Work out the finished part from the listing and answer in its coordinate system (mm). A direction names the side the tool comes from. Coordinates: 2 decimals unless noted, no trailing zeros. Order: outer loops, then holes, each group sorted by start corner. A loop starts at its lowest first (then second) coordinate and runs counter-clockwise, first axis right, second up. Notation, with made-up numbers: M -38,-40 L -27,-40 A6 ccw -27,-31 Z; hole C 60,17 d1. An arc over 180 degrees is marked long. Write item = value, one per line. Start each with the question number.
Q1. Each of these flat-tipped pins is pushed along its axis until it touches: P1, Ø6, axis at x = -25.5, y = 60, coming from the -Z side; P2, Ø3, axis at y = 65.5, z = 7, coming from the -X side; P3, Ø5, axis at y = 123.5, z = 18, coming from the -X side; P4, Ø5, axis at y = 130, z = 4, coming from the +X side. Where does it stop, or does it pass through?
Q2. Find section C-C on x = -15.5. Give the vertices of the cut face in (y, z).
Q3. Find section B-B on y = 122.5. Give the vertices of the cut face in (x, z), and give its area (3 significant figures).
Q4. Straight lines are drawn through the part: line 1 along X through (y, z) = (127, 10); line 2 along Y through (x, z) = (-24, 9); line 3 along X through (y, z) = (125, 8.75). For each, find the intervals that lie inside material, in ascending order.
Q5. Determine the mould class of faces 6 (the flat face through (-37, 94, 25)), 7 (the cylindrical face through (-18.864, 45.315, 12.675)), 8 (the cylindrical face through (-46.17, 166.79, 12.32)), 9 (the cylindrical face through (-56.1, 155.8, 12.3)) for opening direction Y: released by +Y, released by -Y, zero draft, split by the parting line, or undercut.
Q6. A tool of negligible diameter and unlimited length cuts with its end or side. For faces 1 (the flat face through (-36.758, 121.268, 12.325)), 2 (the flat face through (-37.59, 57.57, 12.32)), 3 (the flat face through (-45.76, 86.6, 12.32)), 4 (the flat face through (-33.834, 78, 12)), 5 (the flat face through (-37, 94, 0)), from which of +Z, -Z, +X, -X, +Y, -Y can it reach the whole face along a straight path? Write none if from no direction.
```python
from build123d import *

# Parameters (mm, degrees)
F1_DEPTH  = 25
F2_DEPTH  = 25
F3_R      = 10.0351609687
F4_DEPTH  = 25
F5_W      = 5.021744368
F5_H      = 8.4
F5_W_2    = 5.524914672
F5_H_2    = 8.3
F6_DEPTH  = 28.7
F7_DEPTH  = 31.3
F8_W      = 20.0703219374
F8_H      = 8.3
F8_H_2    = 8.4
F9_DEPTH  = 25
F10_D     = 15
F11_DEPTH = 3
F12_DEPTH = 3
F13_DEPTH = 0.4
F15_DEPTH = 25
F16_R     = 5
F17_R     = 5
F18_R     = 5
F20_DEPTH = 25
F21_R     = 1
F22_DEPTH = 25
F24_DEPTH = 25
F25_R     = 2


with BuildPart() as f1:
    # F0 (on Top) → F1 (new body)
    with BuildSketch(Plane.XY):
        with BuildLine():
            Line((-46.5458918775, 92.7124905365), (-33.8341578848, 67.7643078592))
            Line((-33.8341578848, 67.7643078592), (-33.8341578848, 87.7643078592))
            Line((-33.8341578848, 87.7643078592), (-39.0436032148, 117.3085404495))
            ThreePointArc((-39.0436032148, 117.3085404495), (-50.1493049738, 127.7523979683), (-56.0863416463, 141.7938497088))
            Line((-56.0863416463, 141.7938497088), (-46.5458918775, 92.7124905365))
        make_face()
        Polygon((-26.4959632117, 42.4024048078), (0, 0), (0, 10), (-23.8463668905, 48.162164327), (-33.8341578848, 67.7643078592), (-46.5458918775, 92.7124905365), (-44.6555832012, 78.0426657754), align=None)
    extrude(amount=F1_DEPTH)

    # F0 (on Top) → F2 (join)
    with BuildSketch(Plane.XY):
        Polygon((-26.4959632117, 42.4024048078), (0, 0), (0, 10), (-23.8463668905, 48.162164327), (-33.8341578848, 67.7643078592), (-46.5458918775, 92.7124905365), (-44.6555832012, 78.0426657754), align=None)
        with BuildLine():
            Line((-46.5458918775, 92.7124905365), (-33.8341578848, 67.7643078592))
            Line((-33.8341578848, 67.7643078592), (-33.8341578848, 87.7643078592))
            Line((-33.8341578848, 87.7643078592), (-39.0436032148, 117.3085404495))
            ThreePointArc((-39.0436032148, 117.3085404495), (-50.1493049738, 127.7523979683), (-56.0863416463, 141.7938497088))
            Line((-56.0863416463, 141.7938497088), (-46.5458918775, 92.7124905365))
        make_face()
        with BuildLine():
            ThreePointArc((-51.0571508097, 168.5508889923), (-56.1292788842, 155.6530772369), (-56.0863416463, 141.7938497088))
            ThreePointArc((-56.0863416463, 141.7938497088), (-50.1493049738, 127.7523979683), (-39.0436032148, 117.3085404495))
            ThreePointArc((-39.0436032148, 117.3085404495), (-37.3018340244, 121.656861024), (-34.4069625383, 125.3394376776))
            ThreePointArc((-34.4069625383, 125.3394376776), (-34.1290622054, 125.5985630521), (-33.8452613454, 125.8512122687))
            ThreePointArc((-33.8452613454, 125.8512122687), (-46.0977457681, 142.6841841118), (-42.6035759811, 163.2088788258))
            ThreePointArc((-42.6035759811, 163.2088788258), (-46.2302574516, 166.8295340113), (-51.0571508097, 168.5508889923))
        make_face()
        with BuildLine():
            ThreePointArc((-34.4069625383, 125.3394376776), (-37.3018340244, 121.656861024), (-39.0436032148, 117.3085404495))
            Line((-39.0436032148, 117.3085404495), (-34.4069625383, 125.3394376776))
        make_face()
        with BuildLine():
            ThreePointArc((-46.2700698118, 143.7019396626), (-46.3013690244, 153.8058664235), (-42.6035759811, 163.2088788258))
            ThreePointArc((-42.6035759811, 163.2088788258), (-46.0977457681, 142.6841841118), (-33.8452613454, 125.8512122687))
            ThreePointArc((-33.8452613454, 125.8512122687), (-41.9417428936, 133.4651840398), (-46.2700698118, 143.7019396626))
        make_face()
    extrude(amount=F2_DEPTH)

    # F3 (on Top) → F4 (join)
    with BuildSketch(Plane.XY):
        Circle(F3_R)
    extrude(amount=F4_DEPTH)

    # F5 (on face) → F6 (join)
    with BuildSketch(Plane(origin=(0, 0, 0), x_dir=(0.5299192642, -0.8480480962, 0), z_dir=(-0.8480480962, -0.5299192642, 0))):
        with Locations((-12.5460331527, 4.2)):
            Rectangle(F5_W, F5_H)
        with Locations((-12.7976183047, 20.85)):
            Rectangle(F5_W_2, F5_H_2)
    extrude(amount=F6_DEPTH)

    # F7 (cut, symmetric): faces of the model
    f7_faces = [f1.faces().sort_by_distance(p)[0] for p in [
        (-17.4873152969, 0.9059577124, 20.85),
        (-17.4873152969, 0.9059577124, 4.2),
    ]]
    extrude(f7_faces, amount=F7_DEPTH, both=True, mode=Mode.SUBTRACT)

    # F8 (on face) → F9 (cut)
    with BuildSketch(Plane(origin=(0, 0, 0), x_dir=(0.5299192642, -0.8480480962, 0), z_dir=(-0.8480480962, -0.5299192642, 0))):
        with Locations((0, 20.85)):
            Rectangle(F8_W, F8_H)
        with Locations((0, 4.2)):
            Rectangle(F8_W, F8_H_2)
    extrude(amount=-F9_DEPTH, mode=Mode.SUBTRACT)

    # F10 (through all)
    with Locations(Plane(origin=(0, 0, 0), x_dir=(1, 0, 0), z_dir=(0, 0, -1))):
        with Locations((0, 0)):
            Hole(F10_D / 2)

    # F11 (add): a face of the model
    f11_faces = [f1.faces().sort_by_distance(p)[0] for p in [
        (-15.9068941643, 25.456351981, 12.5),
    ]]
    extrude(f11_faces, amount=F11_DEPTH)

    # F12 (add): a face of the model
    f12_faces = [f1.faces().sort_by_distance(p)[0] for p in [
        (-35.5757732065, 60.2225352916, 12.5),
    ]]
    extrude(f12_faces, amount=F12_DEPTH)

    # F13 (add): a face of the model
    f13_faces = [f1.faces().sort_by_distance(p)[0] for p in [
        (-27.7680353559, 41.6075259115, 12.5),
    ]]
    extrude(f13_faces, amount=F13_DEPTH)

    # F14 (on face) → F15 (join)
    with BuildSketch(Plane.XY.offset(25)):
        with BuildLine():
            ThreePointArc((-44.9484246095, 80.3152745808), (-45.6553028657, 78.1815440804), (-47.3286027738, 76.6806942761))
            Line((-47.3286027738, 76.6806942761), (-44.6555832012, 78.0426657754))
            Line((-44.6555832012, 78.0426657754), (-44.9484246095, 80.3152745808))
        make_face()
        with BuildLine():
            Line((-44.6555832012, 78.0426657754), (-47.3286027738, 76.6806942761))
            Line((-47.3286027738, 76.6806942761), (-29.2321155859, 41.1643384084))
            Line((-29.2321155859, 41.1643384084), (-29.2520752058, 41.1518662536))
            Line((-29.2520752058, 41.1518662536), (-7.8619694055, 6.9205413615))
            Line((-7.8619694055, 6.9205413615), (-0.8238548855, 11.3184434202))
            Line((-0.8238548855, 11.3184434202), (-23.8463668905, 48.162164327))
            Line((-23.8463668905, 48.162164327), (-33.8341578848, 67.7643078592))
            Line((-33.8341578848, 67.7643078592), (-33.8341578848, 87.7643078592))
            Line((-33.8341578848, 87.7643078592), (-39.0436032148, 117.3085404495))
            Line((-39.0436032148, 117.3085404495), (-34.4069625383, 125.3394376776))
            ThreePointArc((-34.4069625383, 125.3394376776), (-34.1290622054, 125.5985630521), (-33.8452613454, 125.8512122687))
            ThreePointArc((-33.8452613454, 125.8512122687), (-46.0541257293, 142.6944106077), (-42.6035759811, 163.2088788258))
            ThreePointArc((-42.6035759811, 163.2088788258), (-46.2302574516, 166.8295340113), (-51.0571508097, 168.5508889923))
            ThreePointArc((-51.0571508097, 168.5508889923), (-56.1292788842, 155.6530772369), (-56.0863416463, 141.7938497088))
            Line((-56.0863416463, 141.7938497088), (-46.5458918775, 92.7124905365))
            Line((-46.5458918775, 92.7124905365), (-45.1575485807, 81.9381904826))
            ThreePointArc((-45.1575485807, 81.9381904826), (-44.9764120983, 81.1365996867), (-44.9484246095, 80.3152745808))
            Line((-44.9484246095, 80.3152745808), (-44.6555832012, 78.0426657754))
        make_face()
    extrude(amount=-F15_DEPTH)

    # F16
    f16_edges = [f1.edges().sort_by_distance(p)[0] for p in [
        (-47.328603, 76.680694, 12.5),
    ]]
    fillet(f16_edges, radius=F16_R)

    # F17
    f17_edges = [f1.edges().sort_by_distance(p)[0] for p in [
        (-33.834158, 67.764308, 12.5),
    ]]
    fillet(f17_edges, radius=F17_R)

    # F18
    f18_edges = [f1.edges().sort_by_distance(p)[0] for p in [
        (-33.834158, 87.764308, 12.5),
    ]]
    fillet(f18_edges, radius=F18_R)

    # F19 (on face) → F20 (join)
    with BuildSketch(Plane.XY.offset(25)):
        with BuildLine():
            Line((-22.2566090978, 45.6180200386), (-20.1369320409, 42.2258276539))
            ThreePointArc((-20.1369320409, 42.2258276539), (-18.8920264045, 45.3620878389), (-22.2566090978, 45.6180200386))
        make_face()
    extrude(amount=-F20_DEPTH)

    # F21 (on face) → F22 (cut)
    with BuildSketch(Plane.XY.offset(25)):
        with Locations((-20.5885408694, 44.3029189806)):
            Circle(F21_R)
    extrude(amount=-F22_DEPTH, mode=Mode.SUBTRACT)

    # F23 (on face) → F24 (cut)
    with BuildSketch(Plane.XY.offset(16.7)):
        Polygon((-21.581498906, -1.6523721461), (-21.581498906, -2.9845223762), (2.6676976122, -15.5032956973), (23.1070481241, 1.1343396036), (-0.8238548855, 11.3184434202), align=None)
    extrude(amount=-F24_DEPTH, mode=Mode.SUBTRACT)

    # F25
    f25_edges = [f1.edges().sort_by_distance(p)[0] for p in [
        (-0.823855, 11.318443, 12.5),
        (-7.861969, 6.920541, 12.5),
    ]]
    fillet(f25_edges, radius=F25_R)


solid = f1.part
```
Findings below:
q1.P1 = through
q1.P2 = -42.4
q1.P3 = -53.02
q1.P4 = -36.25
q2.outline = M 19.14,0 L 34.81,0 L 34.81,25 L 19.14,25 Z
q3.outline = M -52.34,0 L -36.05,0 L -36.05,25 L -52.34,25 Z
q3.area = 407 mm^2
q4.line_1 = -53.21 to -35.58
q4.line_2 = 32.75 to 48.46
q4.line_3 = -52.82 to -34.6
q5.face_6 = zero draft
q5.face_7 = undercut
q5.face_8 = released by +Y
q5.face_9 = split by the parting line
q6.face_1 = +Z, -Z, +X
q6.face_2 = +Z, -Z, -X, -Y
q6.face_3 = +Z, -Z, -X
q6.face_4 = +Z, -Z, +X, +Y
q6.face_5 = -Z, +X, -X, +Y, -Y
